Verification items for this drawing (mm, ordinates from the low corner). A direction names the side the tool comes from. Coordinates: 2 decimals unless noted, no trailing zeros. Write each loop counter-clockwise with the first axis right and the second up, starting at its lowest first coordinate (ties: lowest second). Pieces come first, ordered by that corner, then holes. Notation, with made-up numbers: M 31.5,72 L 40.5,72 A17 ccw 40.5,78 Z; hole C 52.25,68.25 d5. An arc over 180 degrees is marked long. Put each result on its own line as item: value. Start each with the question number.
1) Gauge pin test, flat ends, axial feed: pin 1 (4 mm diameter, centred on x = 5.5, z = 11.5, fed in from -Y); pin 2 (0.8 mm diameter, centred on x = 1, y = 6.5, fed in from +Z); pin 3 (6.5 mm diameter, centred on y = 5.5, z = 8, fed in from +X). Record the tip position at first contact, or that the pin passes through.
2) Cross-section at C-C on x = 2. Record the cut outline in (y, z), plus the area to 3 significant figures.
3) Cross-section at B-B on z = 10. Record the cut outline in (x, y).
4) Scan lines: line 1 along Y through (x, z) = (5.5, 3.55); line 2 along Z through (x, y) = (5.5, 4.85); line 3 along Y through (x, z) = (3.25, 12.25). Record each from-to range of solid material in increasing order.
5) Set-up check for the marked faces 1, 2, 3, 4 and 5: record each of +Z, -Z, +X, -X, +Y, -Y from which the full face is reachable in a straight line by a thin tool's end or side.
6) Cross-section at D-D on z = 4. Record the cut outline in (x, y), plus the area to 3 significant figures.
7) Cross-section at A-A on y = 5.5. Record the cut outline in (x, z), plus the area to 3 significant figures.
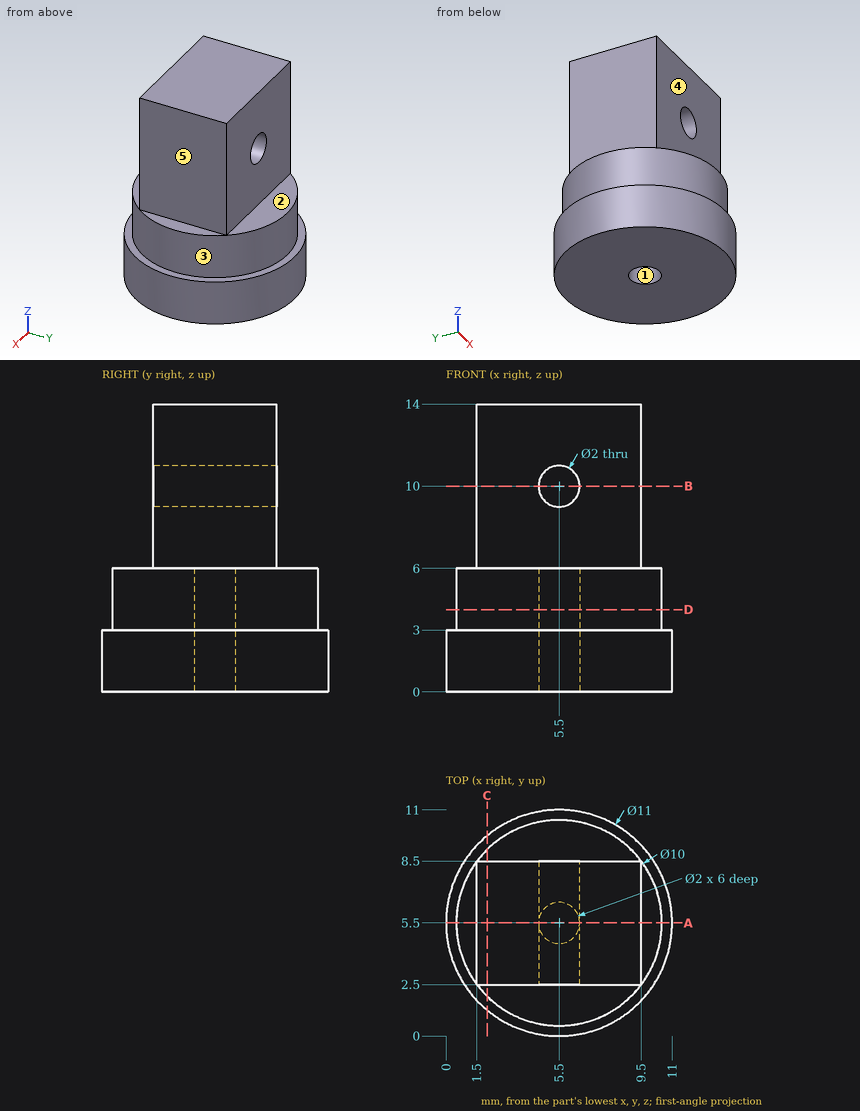
Answer key:
1. pin 1: stops at y = 2.5
1. pin 2: stops at z = 6
1. pin 3: stops at x = 10.5
2. outline: M 1.26,0 L 9.74,0 L 9.74,3 L 9.07,3 L 9.07,6 L 8.5,6 L 8.5,14 L 2.5,14 L 2.5,6 L 1.93,6 L 1.93,3 L 1.26,3 Z
2. area: 94.9 mm²
3. outline: M 1.5,2.5 L 4.5,2.5 L 4.5,8.5 L 1.5,8.5 Z; M 6.5,2.5 L 9.5,2.5 L 9.5,8.5 L 6.5,8.5 Z
4. line 1: y = 0.5 to 4.5, 6.5 to 10.5
4. line 2: z = 6 to 9, 11 to 14
4. line 3: y = 2.5 to 8.5
5. face 1: -Z
5. face 2: +Z, +X, -X, +Y
5. face 3: +Z
5. face 4: +Z, +X, -X, -Y
5. face 5: +Z, +X, +Y, -Y
6. outline: C 5.5,5.5 d10; hole C 5.5,5.5 d2
6. area: 75.4 mm²
7. outline: M 0,0 L 4.5,0 L 4.5,6 L 6.5,6 L 6.5,0 L 11,0 L 11,3 L 10.5,3 L 10.5,6 L 9.5,6 L 9.5,14 L 1.5,14 L 1.5,6 L 0.5,6 L 0.5,3 L 0,3 Z; hole C 5.5,10 d2
7. area: 112 mm²
